Part print with two shaded views. Sizes in mm from the minimum x, y, z corner. A direction names the side the tool comes from. Round coordinates to 2 decimals unless told otherwise and drop trailing zeros. Order: outer loops, then holes, each group sorted by start corner. A loop starts at its lowest first (then second) coordinate and runs counter-clockwise, first axis right, second up. Notation, with made-up numbers: (78.25, 16.25) -> (116.25, 16.25) arc R35 ccw to (116.25, 52.25) -> close; hole circle Ø2 at (-26, -37). An arc over 180 degrees is marked (long way). Put each result on its own line as item: value. Start each with the question number.
Q1. Cut at B-B, the plane z = 11. List the corners of the cut face in (x, y).
Q2. Pull direction X, two halves, no side cores. Call the marked faces 1, 2 and 3: released by +X, released by -X, zero draft, split by the parting line, or undercut.
Q3. Cut at A-A, the plane y = 17.5. List the corners of the cut face in (x, z).
Q4. Flat gauge pins, fed straight in: P1, Ø8, axis at y = 16, z = 8.5, coming from the +X side; P2, Ø2, axis at y = 21, z = 9, coming from the +X side; P3, Ø1.5, axis at y = 29, z = 9, coming from the -X side; P4, Ø8, axis at y = 30.5, z = 5, coming from the +X side. Where does each tip first touch, or does it go through?
Q5. Probe L1, parallel to Y at x = 17.5, z = 3; L2, parallel to Z at x = 33, y = 19.5; L3, parallel to X at y = 12.5, z = 13. List the from-to ranges inside material, lowest first.
Q6. Cut at C-C, the plane z = 1.75. List the corners of the cut face in (x, y).
Q7. 3-axis set-ups, long thin cutter, end or side, ignore diameter. For the marked faces 4 and 5: which of +Z, -Z, +X, -X, +Y, -Y reach the whole face in a straight line?
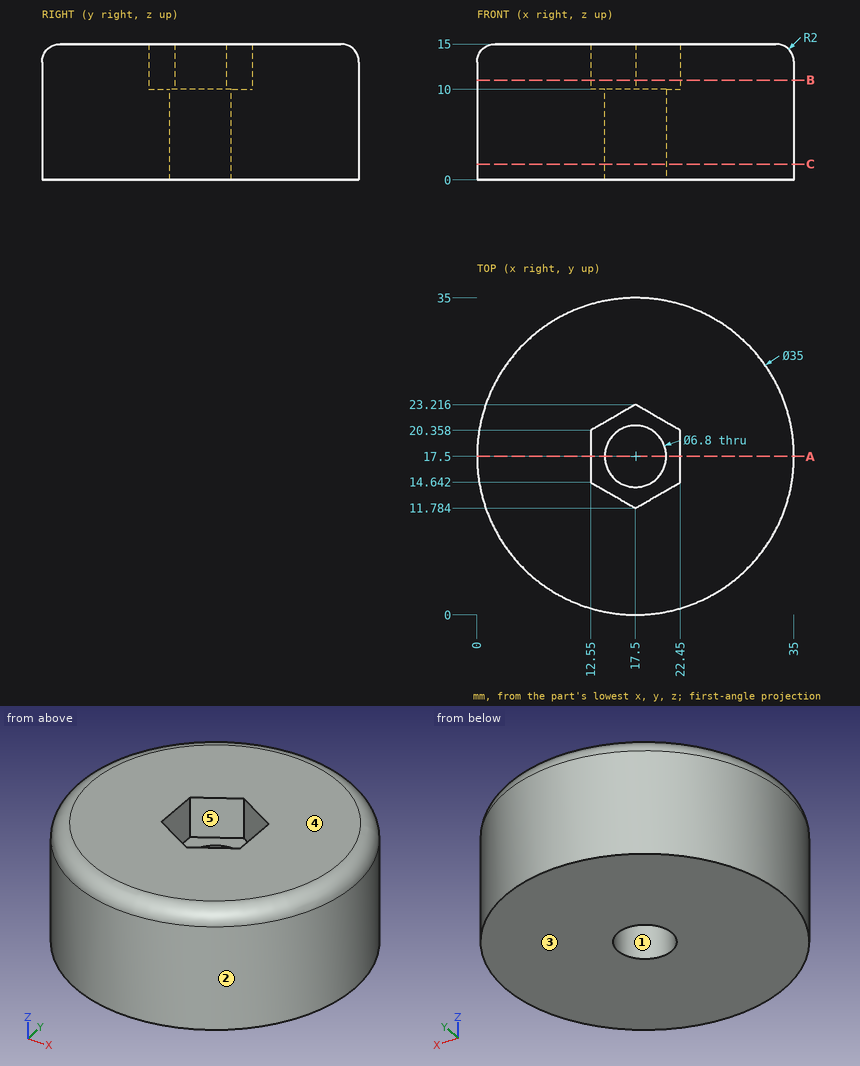
Ans:
1. outline: circle Ø35 at (17.5, 17.5); hole (12.55, 14.64) -> (17.5, 11.78) -> (22.45, 14.64) -> (22.45, 20.36) -> (17.5, 23.22) -> (12.55, 20.36) -> close
2. face 1: undercut
2. face 2: split by the parting line
2. face 3: zero draft
3. outline: (0, 0) -> (14.1, 0) -> (14.1, 10) -> (12.55, 10) -> (12.55, 15) -> (2, 15) arc R2 ccw to (0, 13) -> close; (20.9, 0) -> (35, 0) -> (35, 13) arc R2 ccw to (33, 15) -> (22.45, 15) -> (22.45, 10) -> (20.9, 10) -> close
4. P1: stops at x = 35
4. P2: stops at x = 34.82
4. P3: stops at x = 3.69
4. P4: stops at x = 32.51
5. L1: y = 0 to 14.1, 20.9 to 35
5. L2: z = 0 to 15
5. L3: x = 0.73 to 16.26, 18.74 to 34.27
6. outline: circle Ø35 at (17.5, 17.5); hole circle Ø6.8 at (17.5, 17.5)
7. face 4: +Z, +X, -X, +Y, -Y
7. face 5: +Z
